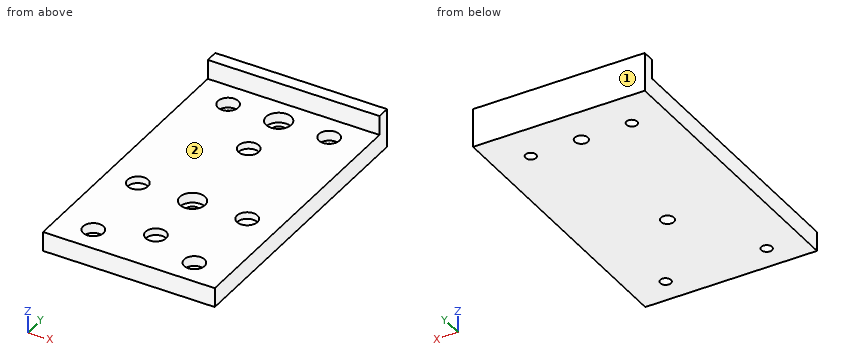
```python
from build123d import *

# Parameters (mm, degrees)
SKETCH1_W                = 68
SKETCH1_H                = 110
SKETCH1_R                = 2.1
SKETCH1_R_2              = 4.05
SKETCH1_R_3              = 2.6
BOSS_EXTRUDE1_DEPTH      = 7.7
SKETCH2_R                = 6.304633146
SKETCH2_R_2              = 7.334333348
SKETCH2_R_3              = 8.114040952
SKETCH2_R_4              = 11.073656437
BOSS_EXTRUDE2_DEPTH      = 5
SKETCH3_R                = 4.05
SKETCH3_R_2              = 5
CUT_EXTRUDE1_DEPTH       = 4
SKETCH4_W                = 68
SKETCH4_H                = 5
BOSS_EXTRUDE3_DEPTH      = 7.7
BOSS_EXTRUDE3_DEPTH_BACK = 7.7


with BuildPart() as part:
    # Sketch1 → Boss-Extrude1 (new body)
    with BuildSketch(Plane.XY):
        Rectangle(SKETCH1_W, SKETCH1_H)
        with Locations((20, 45)):
            Circle(SKETCH1_R, mode=Mode.SUBTRACT)
        with Locations((-20, 45)):
            Circle(SKETCH1_R, mode=Mode.SUBTRACT)
        with Locations((20, -45)):
            Circle(SKETCH1_R, mode=Mode.SUBTRACT)
        with Locations((-20, -45)):
            Circle(SKETCH1_R, mode=Mode.SUBTRACT)
        with Locations((21.650635095, -12.5)):
            Circle(SKETCH1_R_2, mode=Mode.SUBTRACT)
        with Locations((0, 25)):
            Circle(SKETCH1_R_2, mode=Mode.SUBTRACT)
        with Locations((-21.650635095, -12.5)):
            Circle(SKETCH1_R_2, mode=Mode.SUBTRACT)
        with Locations((0, -36.95)):
            Circle(SKETCH1_R_2, mode=Mode.SUBTRACT)
        with Locations((0, 45)):
            Circle(SKETCH1_R_3, mode=Mode.SUBTRACT)
        with Locations((0, -12.5)):
            Circle(SKETCH1_R_3, mode=Mode.SUBTRACT)
    extrude(amount=BOSS_EXTRUDE1_DEPTH)

    # Sketch2 → Boss-Extrude2 (add)
    with BuildSketch(Plane(origin=(0, 0, 0), x_dir=(-1, 0, 0), z_dir=(0, 0, -1))):
        with Locations((-21.650635095, -12.5)):
            Circle(SKETCH2_R)
        with Locations((0, 25)):
            Circle(SKETCH2_R_2)
        with Locations((21.650635095, -12.5)):
            Circle(SKETCH2_R_3)
        with Locations((0, -36.95)):
            Circle(SKETCH2_R_4)
    extrude(amount=-BOSS_EXTRUDE2_DEPTH)

    # Sketch3 → Cut-Extrude1 (cut)
    with BuildSketch(Plane(origin=(0, 0, 7.7), x_dir=(-1, 0, 0), z_dir=(0, 0, -1))):
        with Locations((-20, 45)):
            Circle(SKETCH3_R)
        with Locations((20, 45)):
            Circle(SKETCH3_R)
        with Locations((-20, -45)):
            Circle(SKETCH3_R)
        with Locations((20, -45)):
            Circle(SKETCH3_R)
        with Locations((0, 45)):
            Circle(SKETCH3_R_2)
        with Locations((0, -12.5)):
            Circle(SKETCH3_R_2)
    extrude(amount=CUT_EXTRUDE1_DEPTH, mode=Mode.SUBTRACT)

    # Sketch4 → Boss-Extrude3 (add, two sides)
    with BuildSketch(Plane.XY.offset(7.7)) as boss_extrude3_sk:
        with Locations((0, 57.5)):
            Rectangle(SKETCH4_W, SKETCH4_H)
    extrude(amount=BOSS_EXTRUDE3_DEPTH)
    extrude(boss_extrude3_sk.sketch, amount=-BOSS_EXTRUDE3_DEPTH_BACK)


solid = part.part
```
For this review, take the finished solid that the model builds, in its own axes (mm). Face numbers are marked on the shaded views. A direction names the side the tool comes from. Coordinates: 2 decimals unless noted, no trailing zeros. Order: outer loops, then holes, each group sorted by start corner. A loop starts at its lowest first (then second) coordinate and runs counter-clockwise, first axis right, second up. Notation, with made-up numbers: (10, 39.5) - (30, 39.5) arc R9 cw to (30, 52.5) - close; hole circle Ø3 at (58.25, 74.5). An arc over 180 degrees is marked (long way). Answer as a JSON object with one key per item and string values. Group by question number.
1. For probe 1 along Y at (x, z) = (0, 7.15); probe 2 along X at (y, z) = (45, 1.15); probe 3 along Z at (x, y) = (24, 37), list the stretches that pass through material, from the lowest coordinate up.
2. For the marked faces 1 and 2, list the 3-axis set-ups (+Z, -Z, +X, -X, +Y, -Y) from which the entire face can be reached by the end or side of a thin tool; tool diameter is ignored.
3. We need section C-C on y = -45. State the section outline as (x, z) points.
4. Clearance check with flat-ended pins moving along their axes: P1, Ø8, axis at x = 0.5, y = 45.5, coming from the +Z side; P2, Ø5, axis at x = -21.65, y = -12.5, coming from the -Z side; P3, Ø2.5, axis at x = 22, y = -13, coming from the +Z side; P4, Ø11.5, axis at x = 0, y = 45, coming from the +Z side. State where each tip first meets the part, or that it passes through.
5. We need section B-B on x = 0. Give the number of separate pieces and of enclosed holes in the cut face, then the cut area to 3 significant figures.
6. We need section A-A on y = -12.5. State the section outline as (x, z) points.
Final values:
{
 "1": {"probe 1": "-55 to -41, -32.9 to -17.5, -7.5 to 20.95, 29.05 to 40, 50 to 60", "probe 2": "-34 to -22.1, -17.9 to -2.6, 2.6 to 17.9, 22.1 to 34", "probe 3": "0 to 7.7"},
 "2": {"face 1": "+Z, -Z, +X, -X, +Y", "face 2": "+Z, +X, -X, -Y"},
 "3": {"outline": "(-34, 0) - (-22.1, 0) - (-22.1, 3.7) - (-24.05, 3.7) - (-24.05, 7.7) - (-34, 7.7) - close; (-17.9, 0) - (17.9, 0) - (17.9, 3.7) - (15.95, 3.7) - (15.95, 7.7) - (-15.95, 7.7) - (-15.95, 3.7) - (-17.9, 3.7) - close; (22.1, 0) - (34, 0) - (34, 7.7) - (24.05, 7.7) - (24.05, 3.7) - (22.1, 3.7) - close"},
 "4": {"P1": "z = 3.7", "P2": "z = 0", "P3": "z = 5", "P4": "z = 7.7"},
 "5": {"separate pieces": "3", "enclosed holes": "0", "area": "762 mm²"},
 "6": {"outline": "(-34, 0) - (-2.6, 0) - (-2.6, 3.7) - (-5, 3.7) - (-5, 7.7) - (-17.6, 7.7) - (-17.6, 5) - (-25.7, 5) - (-25.7, 7.7) - (-34, 7.7) - close; (2.6, 0) - (34, 0) - (34, 7.7) - (25.7, 7.7) - (25.7, 5) - (17.6, 5) - (17.6, 7.7) - (5, 7.7) - (5, 3.7) - (2.6, 3.7) - close"}
}
